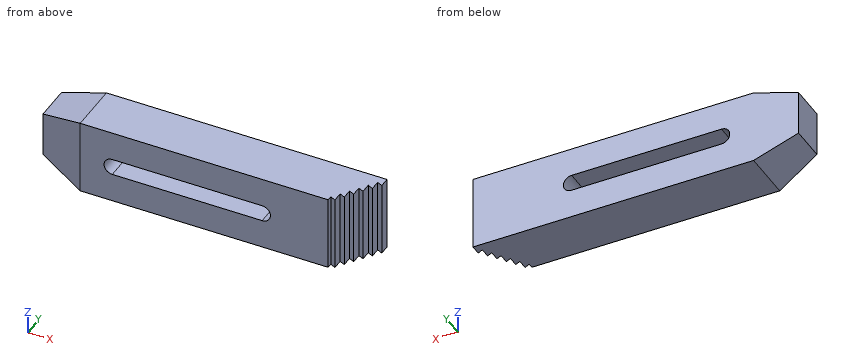
from build123d import *

# Parameters (mm, degrees)
F1_DEPTH   = 25
F1_FACE1_W = 97.703975
F1_FACE1_H = 25
F3_DEPTH   = 25
F4_SIZE2   = 15
F4_SIZE    = 5


with BuildPart() as f1:
    # F0 (on Top) → F1 (new body)
    with BuildSketch(Plane.XY):
        Polygon((-54.298416, 8.472222), (-54.298416, -8.472222), (43.405559, -8.472222), (43.405559, -6.781688), (45.221035, -7.628259), (45.221035, -4.23937), (47.036511, -5.08594), (47.036511, -1.697051), (48.851987, -2.543622), (48.851987, 0.845267), (50.667464, -0.001303), (50.667464, 3.387586), (52.48294, 2.541015), (52.48294, 5.929904), (54.298416, 5.083334), (54.298416, 8.472222), align=None)
    extrude(amount=F1_DEPTH)

    # F2 (on face) + F1_face1 (on face) → F3 (cut)
    with BuildSketch(Plane(origin=(0, 8.472222, 0), x_dir=(-1, 0, 0), z_dir=(0, 1, 0))):
        with BuildLine():
            Line((-21.3955357732, 9.75), (28.6044642268, 9.75))
            ThreePointArc((28.6044642268, 9.75), (31.3544642268, 12.5), (28.6044642268, 15.25))
            Line((28.6044642268, 15.25), (-21.3955357732, 15.25))
            ThreePointArc((-21.3955357732, 15.25), (-24.1455357732, 12.5), (-21.3955357732, 9.75))
        make_face()
    with BuildSketch(Plane(origin=(-5.4464285, -8.472222, 12.5), x_dir=(1, 0, 0), z_dir=(0, -1, 0))):
        Rectangle(F1_FACE1_W, F1_FACE1_H)
    extrude(amount=-F3_DEPTH, dir=(0, 1, 0), mode=Mode.SUBTRACT)

    # F4
    f4_edges = [f1.edges().sort_by_distance(p)[0] for p in [
        (-54.298416, 0, 25),
        (-54.298416, 0, 0),
        (-54.298416, -8.472222, 12.5),
    ]]
    f4_side = f1.faces().sort_by_distance((-54.298416, 0, 12.5))[0]
    chamfer(f4_edges, length=F4_SIZE, length2=F4_SIZE2, reference=f4_side)


solid = f1.part
Build history of the part. All positions in model axes, mm. Coordinates: 2 decimals unless noted, no trailing zeros. Write each loop counter-clockwise with the first axis right and the second up, starting at its lowest first coordinate (ties: lowest second). Pieces come first, ordered by that corner, then holes.
(1) Drill centre lines: line 1 (Z direction, x = 20.5, y = -3.75); line 2 (X direction, y = -3.25, z = 17.5); line 3 (Y direction, x = -43.5, z = 22.5). Where is each one in solid material? Low to high.
(2) Cut at D-D on z = 8.25. List the corners of the cut face in (x, y), and give its area (3 significant figures).
(3) Cut at A-A on z = 12.5. List the corners of the cut face in (x, y), and give its area (3 significant figures).
(4) Cut at C-C on y = 7. List the corners of the cut face in (x, z), and give its area (3 significant figures).
(5) Pin check, flat tips, straight feed: pin 1 Ø1 at (y, z) = (1, 14.5) entering from +X; pin 2 Ø3.5 at (y, z) = (-4, 9) entering from +X; pin 3 Ø2.5 at (y, z) = (-6.5, 18) entering from +X. Stop position of each tip, or through.
(6) Cut at B-B on x = -12.5. List the corners of the cut face in (y, z).
Working result:
1. line 1: z = 0 to 9.75, 15.25 to 25
1. line 2: x = -54.3 to 47.04
1. line 3: y = -7.07 to 8.47
2. outline: (-54.3, -3.47) - (-39.3, -8.47) - (43.41, -8.47) - (43.41, -6.78) - (45.22, -7.63) - (45.22, -4.24) - (47.04, -5.09) - (47.04, -1.7) - (48.85, -2.54) - (48.85, 0.85) - (50.67, 0) - (50.67, 3.39) - (52.48, 2.54) - (52.48, 5.93) - (54.3, 5.08) - (54.3, 8.47) - (-54.3, 8.47) - close
2. area: 1,720 mm2
3. outline: (-54.3, -3.47) - (-39.3, -8.47) - (-31.35, -8.47) - (-31.35, 8.47) - (-54.3, 8.47) - close; (24.15, -8.47) - (43.41, -8.47) - (43.41, -6.78) - (45.22, -7.63) - (45.22, -4.24) - (47.04, -5.09) - (47.04, -1.7) - (48.85, -2.54) - (48.85, 0.85) - (50.67, 0) - (50.67, 3.39) - (52.48, 2.54) - (52.48, 5.93) - (54.3, 5.08) - (54.3, 8.47) - (24.15, 8.47) - close
3. area: 779 mm2
4. outline: (-54.3, 5) - (-39.3, 0) - (54.3, 0) - (54.3, 25) - (-39.3, 25) - (-54.3, 20) - close; hole (-28.6, 9.75) - (21.4, 9.75) arc R2.75 ccw to (21.4, 15.25) - (-28.6, 15.25) arc R2.75 ccw to start
4. area: 2,340 mm2
5. pin 1: stops at x = 50.67
5. pin 2: stops at x = 48.85
5. pin 3: stops at x = 45.22
6. outline: (-8.47, 0) - (8.47, 0) - (8.47, 9.75) - (-8.47, 9.75) - close; (-8.47, 15.25) - (8.47, 15.25) - (8.47, 25) - (-8.47, 25) - close
